from build123d import *

# Parameters (mm, degrees)
T_LE_DE_BASE_PLI_E1_DEPTH               = 100
ESQUISSE9_R                             = 1.5
ENL_V_MAT_EXTRU_1_DEPTH                 = 1
ESQUISSE6_W                             = 38
ESQUISSE6_H                             = 4
PATTE1_DEPTH                            = 1
DIAM_TRE_DU_PER_AGE_3_0_3_1_D           = 3
DIAM_TRE_DU_PER_AGE_3_0_3_1_ON_FACE_2_D = 3


# Sheet-metal steps are written as plain solids
with BuildPart() as part:
    # Esquisse1 → Tôle de base pliée1 (new, symmetric)
    with BuildSketch(Plane.XY):
        with BuildLine():
            Line((27, 0), (30, 129.962877268))
            ThreePointArc((30, 129.962877268), (35.481668982, 158.18527579), (50, 183))
            Line((50, 183), (50.766044443, 182.35721239))
            ThreePointArc((50.766044443, 182.35721239), (36.417352312, 157.832434881), (30.999733682, 129.939799901))
            Line((30.999733682, 129.939799901), (27.999733682, -0.023077367))
            Line((27.999733682, -0.023077367), (27, 0))
        make_face()
    extrude(amount=T_LE_DE_BASE_PLI_E1_DEPTH, both=True)

    # Esquisse9 → Enlèv. mat.-Extru.1 (cut)
    with BuildSketch(Plane(origin=(27.98535443, -0.646000343, 0), x_dir=(0, 0, -1), z_dir=(0.9997336820980194, -0.02307736724014006, 0))):
        with Locations(Location((-95, 45.620586844, 0), (0, 0, 90))):
            Circle(ESQUISSE9_R)
        with Locations(Location((-95, 125.620586844, 0), (0, 0, 90))):
            Circle(ESQUISSE9_R)
        with Locations(Location((0, 125.620586844, 0), (0, 0, 90))):
            Circle(ESQUISSE9_R)
        with Locations(Location((0, 45.620586844, 0), (0, 0, 90))):
            Circle(ESQUISSE9_R)
        with Locations(Location((95, 45.620586844, 0), (0, 0, 270))):
            Circle(ESQUISSE9_R)
        with Locations(Location((95, 125.620586844, 0), (0, 0, 270))):
            Circle(ESQUISSE9_R)
        with BuildLine():
            Line((-69, 5), (-69, 0.623088915))
            Line((-69, 0.623088915), (-100, 0.623088915))
            Line((-100, 0.623088915), (-100, 11))
            Line((-100, 11), (-75, 11))
            ThreePointArc((-75, 11), (-70.757359313, 9.242640687), (-69, 5))
        make_face()
        with BuildLine():
            Line((25, 11), (-25, 11))
            ThreePointArc((-25, 11), (-29.242640687, 9.242640687), (-31, 5))
            Line((-31, 5), (-31, 0.623088915))
            Line((-31, 0.623088915), (31, 0.623088915))
            Line((31, 0.623088915), (31, 5))
            ThreePointArc((31, 5), (29.242640687, 9.242640687), (25, 11))
        make_face()
        with BuildLine():
            Line((100, 11), (75, 11))
            ThreePointArc((75, 11), (70.757359313, 9.242640687), (69, 5))
            Line((69, 5), (69, 0.623088915))
            Line((69, 0.623088915), (100, 0.623088915))
            Line((100, 0.623088915), (100, 11))
        make_face()
    extrude(amount=-ENL_V_MAT_EXTRU_1_DEPTH, mode=Mode.SUBTRACT)

    # Esquisse6 → Patte1 (add)
    with BuildSketch(Plane(origin=(27.98535443, -0.646000343, 0), x_dir=(0, 0, -1), z_dir=(0.9997336820980194, -0.02307736724014006, 0))):
        with Locations((-50, -1.376911085)):
            Rectangle(ESQUISSE6_W, ESQUISSE6_H)
        with Locations((50, -1.376911085)):
            Rectangle(ESQUISSE6_W, ESQUISSE6_H)
    extrude(amount=-PATTE1_DEPTH)

    # Diamètre du perçage Ø3.0 (3)1 (through all)
    with Locations(Plane(origin=(35.938212122, 159.369298961, -95), x_dir=(-0.366675582569, -0.930348868515, 0), z_dir=(-0.930348868515, 0.366675582569, 0))):
        with Locations((0, 0)):
            Hole(DIAM_TRE_DU_PER_AGE_3_0_3_1_D / 2)

    # Diamètre du perçage Ø3.0 (3)1 on face 2 (through all)
    with Locations(Plane(origin=(35.938212122, 159.369298961, 0), x_dir=(-0.366675899022, -0.930348743793, 0), z_dir=(-0.930348743793, 0.366675899022, 0))):
        with Locations((0, 0), (0, 95)):
            Hole(DIAM_TRE_DU_PER_AGE_3_0_3_1_ON_FACE_2_D / 2)


solid = part.part
CAD build for the part. Positions are in the model's coordinates, mm. Coordinates: 2 decimals unless noted, no trailing zeros. Order: outer loops, then holes, each group sorted by start corner. A loop starts at its lowest first (then second) coordinate and runs counter-clockwise, first axis right, second up.
Item 1: Band-saw the part on B-B on x = 44.25. List the corners of the cut face in (y, z), plus the area to 3 significant figures.
Check sheet entries:
outline: (173.48, -100) - (175.31, -100) - (175.31, 100) - (173.48, 100) - close
area: 367 mm2
Item 2: Drill centre lines: L1, parallel to X at y = 8, z = -47; L2, parallel to X at y = 90, z = -12; L3, parallel to Y at x = 44, z = -89.5. Where is each one in solid material? Low to high.
Check sheet entries:
L1: x = 27.18 to 28.18
L2: x = 29.08 to 30.08
L3: y = 173.08 to 174.93
Item 3: Band-saw the part on C-C on y = 30. List the corners of the cut face in (x, z).
Check sheet entries:
outline: (27.69, -100) - (28.69, -100) - (28.69, 100) - (27.69, 100) - close
Item 4: Two-plate mould, pull along Z, no slides. Class faces 1 (the face through (27.71, 8.65, -70.8)), 2 (the face through (27.7, 8.56, -29.29)), 3 (the face through (27.71, 8.65, 70.8)): +Z half, -Z half, draft (parallel to the pull), parting line (faces both ways), or undercut.
Check sheet entries:
face 1: -Z half
face 2: undercut
face 3: +Z half
Item 5: Band-saw the part on D-D on z = 13. List the corners of the cut face in (x, y).
Check sheet entries:
outline: (27.24, 10.37) - (28.24, 10.35) - (31, 129.94) arc R84.58 cw to (50.77, 182.36) - (50, 183) arc R85.58 ccw to (30, 129.96) - close
Item 6: Band-saw the part on A-A on z = 52.5. List the corners of the cut face in (x, y), plus the area to 3 significant figures.
Check sheet entries:
outline: (26.91, -4) - (27.91, -4.02) - (31, 129.94) arc R84.58 cw to (50.77, 182.36) - (50, 183) arc R85.58 ccw to (30, 129.96) - close
area: 191 mm2
Item 7: Pin check, flat tips, straight feed: pin 1 Ø10 at (y, z) = (103.5, -77) entering from +X; pin 2 Ø1.5 at (x, z) = (38.5, -44.5) entering from -Y; pin 3 Ø0.6 at (x, y) = (27, 1) entering from -Z. Stop position of each tip, or through.
Check sheet entries:
pin 1: stops at x = 30.5
pin 2: stops at y = 161.15
pin 3: stops at z = -69
